For this review, take the finished solid that the model builds, in its own axes (mm). A direction names the side the tool comes from. Coordinates: 2 decimals unless noted, no trailing zeros. Loops run counter-clockwise (first coordinate to the right, second up) from the corner with the lowest first, then second, coordinate; pieces in that order, holes last. Notation, with made-up numbers: (30.25, 43) - (74.25, 43) arc R11 cw to (74.25, 54) - close; hole circle Ø8 at (14.5, 30). An arc over 180 degrees is marked (long way). Use one line per item in the form item = value. Start each with the question number.
1. Add section B-B on x = -21. Give the boundary of the cut face in (y, z).
2. To check wall thickness, follow probe 1 along Y at (x, z) = (-18.5, -9.5); probe 2 along X at (y, z) = (-5, -14); probe 3 along Z at (x, y) = (9.5, -47.5). State the ranges of each line that lie inside material, in increasing order.
3. Add section D-D on y = -43. Give the boundary of the cut face in (x, z).
4. Add section C-C on z = -19.75. Give the boundary of the cut face in (x, y).
5. Machinability: for faces 4 (the face through (-25, -24.401, -12)), 5 (the face through (-37.883, -25, -13)), which of the approach directions +Z, -Z, +X, -X, +Y, -Y give a long, thin tool a straight path to every point of the face, cutting with its end or side? Answer none if there is none.
6. Add section A-A on y = -13.5. Give the boundary of the cut face in (x, z).
7. Draft analysis for pull direction X (two halves, no side actions). For faces 1 (the face through (-12, -26, -25.4)), 2 (the face through (12.917, -25, -13)), 3 (the face through (-11.467, -38, -12)), state which applies: +X half, -X half, draft (parallel to the pull), parting line (faces both ways), or undercut.
```python
from build123d import *

# Parameters (mm, degrees)
F0_W     = 25.4
F0_H     = 25.4
F1_DEPTH = 25.4
F2_T     = -1.016
F3_W     = 8.128
F3_H     = 5.08
F4_DEPTH = 25.4


with BuildPart() as f1:
    # F0 (on Top) → F1 (new body)
    with BuildSketch(Plane.XY):
        with Locations((-25.182763, -12.716711)):
            Rectangle(F0_W, F0_H)
    extrude(amount=-F1_DEPTH)

    # F2
    f2_openings = [f1.faces().sort_by_distance(p)[0] for p in [
        (-25.182763, -12.716711, 0),
    ]]
    offset(amount=F2_T, openings=f2_openings)

    # F3 (on Top) → F4 (cut)
    with BuildSketch(Plane.XY):
        with Locations((-24.451679, -12.630123)):
            Rectangle(F3_W, F3_H)
    extrude(amount=-F4_DEPTH, mode=Mode.SUBTRACT)

    # F5: F1 across face


with BuildPart() as f1_1:
    add(f1.part)
    add(f1.part.mirror(Plane(origin=(-12.482763, -12.716711, -12.7), x_dir=(0, 1, 0), z_dir=(1, 0, 0))))

    # F6: F1 across face


with BuildPart() as f1_2:
    add(f1_1.part)
    add(f1_1.part.mirror(Plane(origin=(-12.482763, -25.416711, -12.7), x_dir=(1, 0, 0), z_dir=(0, -1, 0))))


solid = f1_2.part
```
Conclusion:
q1.outline = (-50.82, -25.4) - (-40.74, -25.4) - (-40.74, -24.38) - (-49.8, -24.38) - (-49.8, 0) - (-50.82, 0) - close; (-35.66, -25.4) - (-15.17, -25.4) - (-15.17, -24.38) - (-24.4, -24.38) - (-24.4, 0) - (-26.43, 0) - (-26.43, -24.38) - (-35.66, -24.38) - close; (-10.09, -25.4) - (-0.02, -25.4) - (-0.02, 0) - (-1.03, 0) - (-1.03, -24.38) - (-10.09, -24.38) - close
q2.probe_1 = -50.82 to -49.8, -26.43 to -24.4, -1.03 to -0.02
q2.probe_2 = -37.88 to -36.87, -13.5 to -11.47, 11.9 to 12.92
q2.probe_3 = -25.4 to -24.38
q3.outline = (-37.88, -25.4) - (12.92, -25.4) - (12.92, 0) - (11.9, 0) - (11.9, -24.38) - (-11.47, -24.38) - (-11.47, 0) - (-13.5, 0) - (-13.5, -24.38) - (-36.87, -24.38) - (-36.87, 0) - (-37.88, 0) - close
q4.outline = (-37.88, -50.82) - (12.92, -50.82) - (12.92, -0.02) - (-37.88, -0.02) - close; hole (-36.87, -49.8) - (-13.5, -49.8) - (-13.5, -26.43) - (-36.87, -26.43) - close; hole (-36.87, -24.4) - (-13.5, -24.4) - (-13.5, -1.03) - (-36.87, -1.03) - close; hole (-11.47, -49.8) - (11.9, -49.8) - (11.9, -26.43) - (-11.47, -26.43) - close; hole (-11.47, -24.4) - (11.9, -24.4) - (11.9, -1.03) - (-11.47, -1.03) - close
q5.face_4 = +Z
q5.face_5 = +Z, -Z, -X, +Y, -Y
q6.outline = (-37.88, -25.4) - (-28.52, -25.4) - (-28.52, -24.38) - (-36.87, -24.38) - (-36.87, 0) - (-37.88, 0) - close; (-20.39, -25.4) - (-4.58, -25.4) - (-4.58, -24.38) - (-11.47, -24.38) - (-11.47, 0) - (-13.5, 0) - (-13.5, -24.38) - (-20.39, -24.38) - close; (3.55, -25.4) - (12.92, -25.4) - (12.92, 0) - (11.9, 0) - (11.9, -24.38) - (3.55, -24.38) - close
q7.face_1 = draft
q7.face_2 = +X half
q7.face_3 = undercut
